For this review, take the finished solid that the model builds, in its own axes (mm). A direction names the side the tool comes from. Round coordinates to 2 decimals unless told otherwise and drop trailing zeros. Loops run counter-clockwise (first coordinate to the right, second up) from the corner with the lowest first, then second, coordinate; pieces in that order, holes last.
1. Draft analysis for pull direction Z (two halves, no side actions). For faces 6 (the flat face through (253.49, 10, -140)), 7 (the flat face through (403.49, 148, -220)), state which applies: released by +Z, released by -Z, zero draft, split by the parting line, or undercut.
2. To check wall thickness, follow line 1 along Y through (x, z) = (-3.5, -355). State the ranges of the line that lie inside material, in increasing order.
3. Tool access review of faces 1 (the flat face through (-171.51, 149, -11)), 2 (the flat face through (414, 260, -603)), 3 (the flat face through (439, 20, -603)), 4 (the flat face through (-1.51, 10, -445)), 5 (the flat face through (-182, 165, -523)): name each direction out of +Z, -Z, +X, -X, +Y, -Y from which nothing blocks a thin tool from reaching the whole face with its end or side.
4. Consider section A-A on z = -491. State the section outline as (x, y) points, then the cut area to 3 significant figures.
5. Clearance check with flat-ended pins moving along their axes: pin 1 Ø10 at (y, z) = (13.5, -413.5) entering from -X; pin 2 Ø22 at (x, z) = (411.5, -183.5) entering from -Y; pin 3 Ø10 at (x, z) = (-179, 14.5) entering from +Y; pin 4 Ø12 at (x, z) = (7.5, -225) entering from +Y. State where each tip first meets the part, or that it passes through.
6. Consider section B-B on y = 442.5. State the section outline as (x, z) points, then the cut area to 3 significant figures.
7. Consider section D-D on y = 178.5. State the section outline as (x, z) points, then the cut area to 3 significant figures.
8. Consider section C-C on x = 278.5. State the section outline as (y, z) points.
from build123d import *

# Parameters (mm, degrees)
SKETCH_1_W          = 235
SKETCH_1_H          = 600
EXTRUDE_1_DEPTH     = 20
EXTRUDE_4_DEPTH     = 20
SKETCH_6_W          = 640
SKETCH_6_H          = 20
EXTRUDE_6_DEPTH     = 20
SKETCH1_W           = 320
SKETCH1_H           = 20
CUT_EXTRUDE1_DEPTH  = 20
SKETCH2_W           = 515
SKETCH2_H           = 20
EXTRUDE1_DEPTH      = 20
SKETCH3_W           = 20
SKETCH3_H           = 20
BOSS_EXTRUDE1_DEPTH = 285


with BuildPart() as part:
    # 草图1 → 凸台-拉伸1 (new body)
    with BuildSketch(Plane(origin=(0, 0, 0), x_dir=(1, 0, 0), z_dir=(0, 1, 0))):
        Polygon((-221.510078765, -7.502951786), (-21.510078765, -7.502951786), (-21.510078765, 592.497048214), (-221.510078765, 592.497048214), (-221.510078765, 612.497048214), (453.489921235, 612.497048214), (453.489921235, 592.497048214), (253.489921235, 592.497048214), (253.489921235, -7.502951786), (453.489921235, -7.502951786), (453.489921235, -27.502951786), (-221.510078765, -27.502951786), align=None)
        with Locations((115.989921235, 292.497048214)):
            Rectangle(SKETCH_1_W, SKETCH_1_H, mode=Mode.SUBTRACT)
    extrude(amount=EXTRUDE_1_DEPTH)

    # 草图2 → 凸台-拉伸4 (add)
    with BuildSketch(Plane.ZY.offset(191.510078765)):
        Polygon((27.502951786, 20), (7.502951786, 20), (7.502951786, 165), (7.502951786, 260), (27.502951786, 260), align=None)
        Polygon((-592.497048214, 260), (-592.497048214, 165), (-592.497048214, 20), (-612.497048214, 20), (-612.497048214, 260), align=None)
    extrude_4 = extrude(amount=-EXTRUDE_4_DEPTH)

    # 镜向3: 凸台-拉伸4 across plane
    add(extrude_4.mirror(Plane(origin=(115.989921235, 0, 0), x_dir=(0, 0, 1), z_dir=(1, 0, 0))))

    # 草图6 → 凸台-拉伸6 (add)
    with BuildSketch(Plane.ZY.offset(191.510078765)):
        with Locations((-292.497048214, 155)):
            Rectangle(SKETCH_6_W, SKETCH_6_H)
    extrude_6 = extrude(amount=-EXTRUDE_6_DEPTH)

    # 镜向6: 凸台-拉伸6 across plane
    add(extrude_6.mirror(Plane(origin=(115.989921235, 0, 0), x_dir=(0, 0, 1), z_dir=(1, 0, 0))))

    # Sketch1 → Cut-Extrude1 (cut)
    with BuildSketch(Plane.ZY.offset(191.510078765)):
        with Locations((-292.497048214, 155)):
            Rectangle(SKETCH1_W, SKETCH1_H)
    extrude(amount=-CUT_EXTRUDE1_DEPTH, mode=Mode.SUBTRACT)

    # Sketch2 → Extrude1 (add)
    with BuildSketch(Plane(origin=(0, 0, 0), x_dir=(-1, 0, 0), z_dir=(0, -1, 0))):
        with Locations((-115.989921235, 292.497048214)):
            Rectangle(SKETCH2_W, SKETCH2_H)
    extrude(amount=-EXTRUDE1_DEPTH)

    # Sketch3 → Boss-Extrude1 (add)
    with BuildSketch(Plane(origin=(0, 260, 0), x_dir=(1, 0, 0), z_dir=(0, 1, 0))):
        with Locations((-181.510078765, 602.497048214)):
            Rectangle(SKETCH3_W, SKETCH3_H)
        with Locations((413.489921235, -17.502951786)):
            Rectangle(SKETCH3_W, SKETCH3_H)
    extrude(amount=BOSS_EXTRUDE1_DEPTH)


solid = part.part
Resolved:
1. face 6: undercut
1. face 7: zero draft
2. line 1: y = 0 to 20
3. face 1: +Z, -Z, +Y
3. face 2: -Z, +X, +Y
3. face 3: +Z, -Z, +X, +Y
3. face 4: +Y, -Y
3. face 5: +X, -X, +Y
4. outline: (-191.51, 145) - (-171.51, 145) - (-171.51, 165) - (-191.51, 165) - close; (-21.51, 0) - (-1.51, 0) - (-1.51, 20) - (-21.51, 20) - close; (233.49, 0) - (253.49, 0) - (253.49, 20) - (233.49, 20) - close; (403.49, 145) - (423.49, 145) - (423.49, 165) - (403.49, 165) - close
4. area: 1,600 mm2
5. pin 1: stops at x = -21.51
5. pin 2: stops at y = 145
5. pin 3: stops at y = 260
5. pin 4: passes through
6. outline: (-191.51, -612.5) - (-171.51, -612.5) - (-171.51, -592.5) - (-191.51, -592.5) - close; (403.49, 7.5) - (423.49, 7.5) - (423.49, 27.5) - (403.49, 27.5) - close
6. area: 800 mm2
7. outline: (-191.51, -612.5) - (-171.51, -612.5) - (-171.51, -592.5) - (-191.51, -592.5) - close; (-191.51, 7.5) - (-171.51, 7.5) - (-171.51, 27.5) - (-191.51, 27.5) - close; (403.49, -612.5) - (423.49, -612.5) - (423.49, -592.5) - (403.49, -592.5) - close; (403.49, 7.5) - (423.49, 7.5) - (423.49, 27.5) - (403.49, 27.5) - close
7. area: 1,600 mm2
8. outline: (0, -612.5) - (20, -612.5) - (20, -592.5) - (0, -592.5) - close; (0, -302.5) - (20, -302.5) - (20, -282.5) - (0, -282.5) - close; (0, 7.5) - (20, 7.5) - (20, 27.5) - (0, 27.5) - close
